The model under review builds one solid part; all positions refer to its coordinate system, in mm. A direction names the side the tool comes from. Round coordinates to 2 decimals unless told otherwise and drop trailing zeros. Write each loop counter-clockwise with the first axis right and the second up, starting at its lowest first coordinate (ties: lowest second). Pieces come first, ordered by that corner, then holes. Notation, with made-up numbers: (59, 84.5) - (78, 84.5) arc R29 cw to (78, 117.5) - close; hole circle Ø7 at (-21, 43.5). An arc over 180 degrees is marked (long way). Use one line per item in the form item = value.
from build123d import *

# Parameters (mm, degrees)
F0_R      = 75.565
F1_DEPTH  = 101.6
F2_DEPTH  = 127
F3_R      = 38.1
F4_DEPTH  = 127
F5_R      = 75.565
F6_DEPTH  = 127
F7_R      = 73.914
F8_DEPTH  = 228.6010001
F9_R      = 73.914
F10_DEPTH = 127.001
F11_R     = 36.449
F12_DEPTH = 62.6989799529


with BuildPart() as f1:
    # F0 (on Top) → F1 (new body)
    with BuildSketch(Plane.XY):
        Circle(F0_R)
    extrude(amount=F1_DEPTH)

    # F0 (on Top) → F2 (join)
    with BuildSketch(Plane.XY):
        Circle(F0_R)
    extrude(amount=-F2_DEPTH)

    # F3 (on Front) → F4 (join)
    with BuildSketch(Plane.XZ):
        Circle(F3_R)
    extrude(amount=F4_DEPTH)

    # F5 (on Right) → F6 (join)
    with BuildSketch(Plane.YZ):
        Circle(F5_R)
    extrude(amount=F6_DEPTH)

    # F7 (on face) → F8 (cut, through all)
    with BuildSketch(Plane.XY.offset(101.6)):
        Circle(F7_R)
    extrude(amount=-F8_DEPTH, mode=Mode.SUBTRACT)

    # F9 (on face) → F10 (cut, through all)
    with BuildSketch(Plane.YZ.offset(127)):
        Circle(F9_R)
    extrude(amount=-F10_DEPTH, mode=Mode.SUBTRACT)

    # F11 (on face) → F12 (cut, through all)
    with BuildSketch(Plane.XZ.offset(127)):
        Circle(F11_R)
    extrude(amount=-F12_DEPTH, mode=Mode.SUBTRACT)


solid = f1.part
(1) Add section A-A on x = -61.5. Write out the cut boundary in (y, z).
Geometry results:
outline = (-43.91, -127) - (-41, -127) - (-41, 101.6) - (-43.91, 101.6) - close; (41, -127) - (43.91, -127) - (43.91, 101.6) - (41, 101.6) - close
(2) Insertion check: P1, Ø1, axis at x = -18.5, z = 67.5, coming from the -Y side; P2, Ø12, axis at x = -23.5, z = 57.5, coming from the +Y side; P3, Ø2, axis at y = -18.5, z = 58.5, coming from the +X side. Each pin has a flat end and moves straight along its axis. Give the tip position at first contact, or say it passes through.
Geometry results:
P1 = -73.39
P2 = 73.51
P3 = -71.3
(3) The part is to be moulded in two halves that separate along Y. For faces 4 (the flat face through (127, 16.4, -72.4)), 5 (the flat face through (20, -127, -31)), 6 (the cylindrical face through (-73.843, 3.25, -11.1)), 7 (the cylindrical face through (-75.492, 3.322, -11.1)), say which applies: +Y half, -Y half, draft (parallel to the pull), parting line (faces both ways), or undercut.
Geometry results:
face_4 = draft
face_5 = -Y half
face_6 = undercut
face_7 = parting line
(4) Add section B-B on y = -16. Write out the cut boundary in (x, z).
Geometry results:
outline = (-73.85, -127) - (-72.16, -127) - (-72.16, 101.6) - (-73.85, 101.6) - close; (72.16, -127) - (73.85, -127) - (73.85, -73.85) - (127, -73.85) - (127, -72.16) - (72.16, -72.16) - close; (72.16, 72.16) - (127, 72.16) - (127, 73.85) - (73.85, 73.85) - (73.85, 101.6) - (72.16, 101.6) - close
(5) To check wall thickness, follow L1, parallel to Y at x = 52, z = 3; L2, parallel to Y at x = 2.5, z = -57.5; L3, parallel to X at y = -91, z = 0. State the ranges of each line that lie inside material, in increasing order.
Geometry results:
L1 = -75.51 to -73.85, 73.85 to 75.51
L2 = -75.52 to -73.87, 73.87 to 75.52
L3 = -38.1 to -36.45, 36.45 to 38.1
(6) Add section C-C on z = -9. Write out the cut boundary in (x, y) (3 decimals), then the cut area to 3 significant figures.
Geometry results:
outline = (-37.022, -127) - (-35.32, -127) - (-35.32, -64.929) arc R73.914 cw to (9, 73.364) - (127, 73.364) - (127, 75.027) - (9, 75.027) arc R75.565 ccw to (-37.022, -65.875) - close; (35.32, -127) - (37.022, -127) - (37.022, -75.027) - (127, -75.027) - (127, -73.364) - (35.32, -73.364) - close
area = 882 mm2
(7) Machinability: for faces 1 (the cylindrical face through (-28.925, -96.09, -22.179)), 2 (the flat face through (16.4, -72.4, -127)), 3 (the cylindrical face through (90.833, 69.803, -28.942)), which of the approach directions +Z, -Z, +X, -X, +Y, -Y give a long, thin tool a straight path to every point of the face, cutting with its end or side? Answer none if there is none.
Geometry results:
face_1 = -Y
face_2 = -Z, +X, -X, +Y, -Y
face_3 = +X
